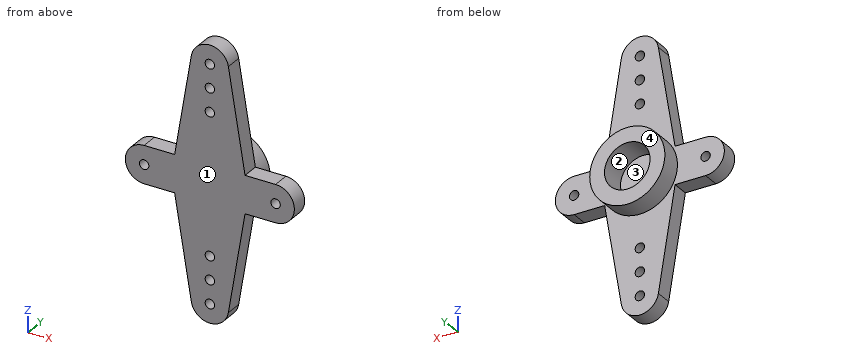
```python
from build123d import *

# Parameters (mm, degrees)
BOSS_EXTRUDE1_DEPTH = 1.8
SKETCH2_R           = 4
BOSS_EXTRUDE2_DEPTH = 2.2
SKETCH3_R           = 2.425
CUT_EXTRUDE1_DEPTH  = 2.8
SKETCH4_R           = 0.5
CUT_EXTRUDE2_DEPTH  = 2.8


with BuildPart() as part:
    # Sketch1 → Boss-Extrude1 (new body)
    with BuildSketch(Plane(origin=(0, 0, 0), x_dir=(1, 0, 0), z_dir=(0, 1, 0))):
        with BuildLine():
            Line((-3.75, 2), (-1.973597307, 12.8239038))
            ThreePointArc((-1.973597307, 12.8239038), (0, 14.5), (1.973597307, 12.8239038))
            Line((1.973597307, 12.8239038), (3.75, 2))
            Line((3.75, 2), (7, 2))
            ThreePointArc((7, 2), (9, 0), (7, -2))
            Line((7, -2), (3.75, -2))
            Line((3.75, -2), (1.973597307, -12.8239038))
            ThreePointArc((1.973597307, -12.8239038), (0, -14.5), (-1.973597307, -12.8239038))
            Line((-1.973597307, -12.8239038), (-3.75, -2))
            Line((-3.75, -2), (-7, -2))
            ThreePointArc((-7, -2), (-9, 0), (-7, 2))
            Line((-7, 2), (-3.75, 2))
        make_face()
    extrude(amount=BOSS_EXTRUDE1_DEPTH)

    # Sketch2 → Boss-Extrude2 (add)
    with BuildSketch(Plane(origin=(0, 1.8, 0), x_dir=(1, 0, 0), z_dir=(0, 1, 0))):
        Circle(SKETCH2_R)
    extrude(amount=BOSS_EXTRUDE2_DEPTH)

    # Sketch3 → Cut-Extrude1 (cut)
    with BuildSketch(Plane(origin=(0, 4, 0), x_dir=(1, 0, 0), z_dir=(0, 1, 0))):
        Circle(SKETCH3_R)
    extrude(amount=-CUT_EXTRUDE1_DEPTH, mode=Mode.SUBTRACT)

    # Sketch4 → Cut-Extrude2 (cut, through all)
    with BuildSketch(Plane(origin=(0, 1.8, 0), x_dir=(1, 0, 0), z_dir=(0, 1, 0))):
        with Locations((-7, 0)):
            Circle(SKETCH4_R)
        with Locations((7, 0)):
            Circle(SKETCH4_R)
        with Locations((0, 7.5)):
            Circle(SKETCH4_R)
        with Locations((0, -7.5)):
            Circle(SKETCH4_R)
        with Locations((0, 10)):
            Circle(SKETCH4_R)
        with Locations((0, 12.5)):
            Circle(SKETCH4_R)
        with Locations((0, -10)):
            Circle(SKETCH4_R)
        with Locations((0, -12.5)):
            Circle(SKETCH4_R)
    extrude(amount=-CUT_EXTRUDE2_DEPTH, mode=Mode.SUBTRACT)


solid = part.part
```
Geometry: final body of the model. Coordinates: model frame, mm. Face numbers are marked on the shaded views. A direction names the side the tool comes from. Give positions to 0.01 mm unless a question says otherwise; leave off trailing zeros. Order: outer loops, then holes, each group sorted by start corner. A loop starts at its lowest first (then second) coordinate and runs counter-clockwise, first axis right, second up. Notation, with made-up numbers: M 2,38.25 L 11,38.25 A8 ccw 11,47.25 Z; hole C -14.75,50 d4. An arc over 180 degrees is marked long. Answer as CSV lines item,"result". Start each with the question number.
1) Cut plane A-A (z = 12.5). Output: boundary loops of the cut face in (x, y).
2) Cut plane C-C (y = 3.4). Output: boundary loops of the cut face in (x, z) (3 decimals).
3) Set-up query: the marked faces 1 and 2. Return all of +Z, -Z, +X, -X, +Y, -Y with unobstructed straight access to the full face (end or side cutting, diameter ignored); none if empty.
4) First-contact query: P1, Ø1, axis at x = -6.5, y = 1, coming from the +Z side; P2, Ø0.9, axis at x = 6, y = 1.5, coming from the -Z side; P3, Ø8, axis at x = -6, z = -5.5, coming from the +Y side. Flat tips, straight axial feed; report the tip coordinate or a pass-through.
5) Line query: line 1 (X direction, y = 0.75, z = 0); line 2 (X direction, y = 1.45, z = 0) (3 decimals); line 3 (Y direction, x = 3, z = 6.25). Output: solid intervals per line, ascending. Write a range as from..to.
6) Cut plane D-D (z = 3.25). Output: boundary loops of the cut face in (x, y).
7) Mould query, pull axis X, two halves, no side actions, for the marked faces 3 and 4. Classes: +X half, -X half, draft (parallel to the pull), parting line (faces both ways), or undercut.
8) Cut plane B-B (y = 0.9). State how many separate pieces and enclosed holes the cut face has, then the cut area to 3 significant figures.
Findings below:
1,outline,"M -2.03,0 L -0.5,0 L -0.5,1.8 L -2.03,1.8 Z; M 0.5,0 L 2.03,0 L 2.03,1.8 L 0.5,1.8 Z"
2,outline,"C 0,0 d8; hole C 0,0 d4.85"
3,face 1,"+Z, -Z, +X, -X, -Y"
3,face 2,"+Y"
4,P1,"stops at z = 2"
4,P2,"stops at z = -2"
4,P3,"stops at y = 1.8"
5,line 1,"x = -9..-7.5, -6.5..6.5, 7.5..9"
5,line 2,"x = -9..-7.5, -6.5..-2.425, 2.425..6.5, 7.5..9"
5,line 3,"y = 0..1.8"
6,outline,"M -3.54,0 L 3.54,0 L 3.54,1.8 L 2.33,1.8 L 2.33,4 L -2.33,4 L -2.33,1.8 L -3.54,1.8 Z"
7,face 3,"undercut"
7,face 4,"draft"
8,separate pieces,"1"
8,enclosed holes,"8"
8,area,"196 mm²"
